Source: CAD feature listing. Evaluate the final solid. Frame: model axes, mm. Give positions to 0.01 mm unless a question says otherwise; leave off trailing zeros. Write each loop counter-clockwise with the first axis right and the second up, starting at its lowest first coordinate (ties: lowest second). Pieces come first, ordered by that corner, then holes. Notation, with made-up numbers: (50, 32.5) -> (107, 32.5) arc R19 cw to (107, 53.5) -> close; hole circle Ø11 at (75, 21). An arc over 180 degrees is marked (long way). Use a Markdown table: item, result. Add a question column.
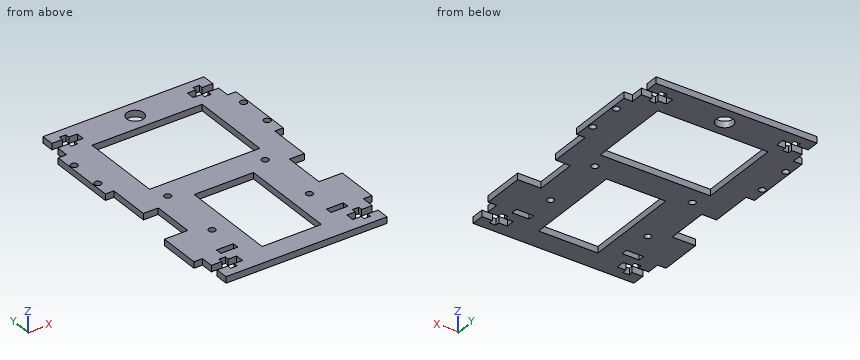
```python
from build123d import *

# Parameters (mm, degrees)
SKETCH_1_W      = 8
SKETCH_1_H      = 3
SKETCH_1_R      = 1.6
SKETCH_1_W_2    = 28
SKETCH_1_H_2    = 46
SKETCH_1_W_3    = 52
SKETCH_1_H_3    = 39
SKETCH_1_R_2    = 4
EXTRUDE_1_DEPTH = 3


with BuildPart() as part:
    # 草图1 → 凸台-拉伸1 (new body)
    with BuildSketch(Plane.XY):
        Polygon((-42, 70), (-42, 54), (-42, 38), (-38, 38), (-38, 18), (-31, 18), (-31, -2), (-38, -2), (-42, -2), (-42, -22), (-38, -22), (-38, -28), (-33, -28), (-33, -26), (-30, -26), (-30, -28), (-26, -28), (-26, -32), (-30, -32), (-30, -34), (-33, -34), (-33, -32), (-38, -32), (-38, -38), (38, -38), (38, -32), (33, -32), (33, -34), (30, -34), (30, -32), (26, -32), (26, -28), (30, -28), (30, -26), (33, -26), (33, -28), (38, -28), (38, -22), (42, -22), (42, -2), (38, -2), (31, -2), (31, 18), (38, 18), (38, 38), (42, 38), (42, 54), (42, 70), (38, 70), (38, 76), (33, 76), (33, 74), (30, 74), (30, 76), (26, 76), (26, 80), (30, 80), (30, 82), (33, 82), (33, 80), (38, 80), (38, 86), (-38, 86), (-38, 80), (-33, 80), (-33, 82), (-30, 82), (-30, 80), (-26, 80), (-26, 76), (-30, 76), (-30, 74), (-33, 74), (-33, 76), (-38, 76), (-38, 70), align=None)
        with Locations((-26, -21.5)):
            Rectangle(SKETCH_1_W, SKETCH_1_H, mode=Mode.SUBTRACT)
        with Locations((-23, -7)):
            Circle(SKETCH_1_R, mode=Mode.SUBTRACT)
        with Locations((-23, 23)):
            Circle(SKETCH_1_R, mode=Mode.SUBTRACT)
        with Locations((26, -21.5)):
            Rectangle(SKETCH_1_W, SKETCH_1_H, mode=Mode.SUBTRACT)
        with Locations((0, -5)):
            Rectangle(SKETCH_1_W_2, SKETCH_1_H_2, mode=Mode.SUBTRACT)
        with Locations((23, -7)):
            Circle(SKETCH_1_R, mode=Mode.SUBTRACT)
        with Locations((23, 23)):
            Circle(SKETCH_1_R, mode=Mode.SUBTRACT)
        with Locations((-40, 46)):
            Circle(SKETCH_1_R, mode=Mode.SUBTRACT)
        with Locations((0, 50.5)):
            Rectangle(SKETCH_1_W_3, SKETCH_1_H_3, mode=Mode.SUBTRACT)
        with Locations((-40, 62)):
            Circle(SKETCH_1_R, mode=Mode.SUBTRACT)
        with Locations((40, 46)):
            Circle(SKETCH_1_R, mode=Mode.SUBTRACT)
        with Locations((0, 78)):
            Circle(SKETCH_1_R_2, mode=Mode.SUBTRACT)
        with Locations((40, 62)):
            Circle(SKETCH_1_R, mode=Mode.SUBTRACT)
    extrude(amount=EXTRUDE_1_DEPTH)


solid = part.part
```
(1) Cut plane B-B on x = 0. Return the cut outline in (y, z), then the cut area to 3 significant figures.
(2) Cut plane C-C on y = -4. Return the cut outline in (x, z), then the cut area to 3 significant figures.
(3) Cut plane D-D on y = 46. Return the cut outline in (x, z).
(4) Cut plane A-A on y = 23. Return the cut outline in (x, z).
(5) Material intervals for L1, parallel to Y at x = 0, z = 2.25; L2, parallel to Y at x = -6, z = 2.9; L3, parallel to Y at x = -21, z = 2.8, sorted ascending.
(6) First-contact query: pin 1 Ø0.9 at (y, z) = (83, 1) entering from -X; pin 2 Ø0.9 at (y, z) = (-29.5, 1) entering from -X; pin 3 Ø1.5 at (y, z) = (-36.5, 1.5) entering from +X. Flat tips, straight axial feed; report the tip coordinate or a pass-through.
Output:
| question | item | result |
|---|---|---|
| 1 | outline | (-38, 0) -> (-28, 0) -> (-28, 3) -> (-38, 3) -> close; (18, 0) -> (31, 0) -> (31, 3) -> (18, 3) -> close; (70, 0) -> (74, 0) -> (74, 3) -> (70, 3) -> close; (82, 0) -> (86, 0) -> (86, 3) -> (82, 3) -> close |
| 1 | area | 93.0 mm^2 |
| 2 | outline | (-42, 0) -> (-14, 0) -> (-14, 3) -> (-42, 3) -> close; (14, 0) -> (42, 0) -> (42, 3) -> (14, 3) -> close |
| 2 | area | 168 mm^2 |
| 3 | outline | (-42, 0) -> (-41.6, 0) -> (-41.6, 3) -> (-42, 3) -> close; (-38.4, 0) -> (-26, 0) -> (-26, 3) -> (-38.4, 3) -> close; (26, 0) -> (38.4, 0) -> (38.4, 3) -> (26, 3) -> close; (41.6, 0) -> (42, 0) -> (42, 3) -> (41.6, 3) -> close |
| 4 | outline | (-38, 0) -> (-24.6, 0) -> (-24.6, 3) -> (-38, 3) -> close; (-21.4, 0) -> (21.4, 0) -> (21.4, 3) -> (-21.4, 3) -> close; (24.6, 0) -> (38, 0) -> (38, 3) -> (24.6, 3) -> close |
| 5 | L1 | -38 to -28, 18 to 31, 70 to 74, 82 to 86 |
| 5 | L2 | -38 to -28, 18 to 31, 70 to 86 |
| 5 | L3 | -38 to 31, 70 to 86 |
| 6 | pin 1 | x = -38 |
| 6 | pin 2 | x = -26 |
| 6 | pin 3 | x = 38 |
